Print and shaded views of the part. All mm, measured from the part's lowest x, y and z. A direction names the side the tool comes from. Round coordinates to 2 decimals unless told otherwise and drop trailing zeros. Loops run counter-clockwise (first coordinate to the right, second up) from the corner with the lowest first, then second, coordinate; pieces in that order, holes last. Notation, with made-up numbers: (-14.5, -27.75) - (5.5, -27.75) arc R15 cw to (5.5, -5.75) - close; hole circle Ø11 at (4.25, -33.75). An arc over 180 degrees is marked (long way). Use one line per item in the form item = value.
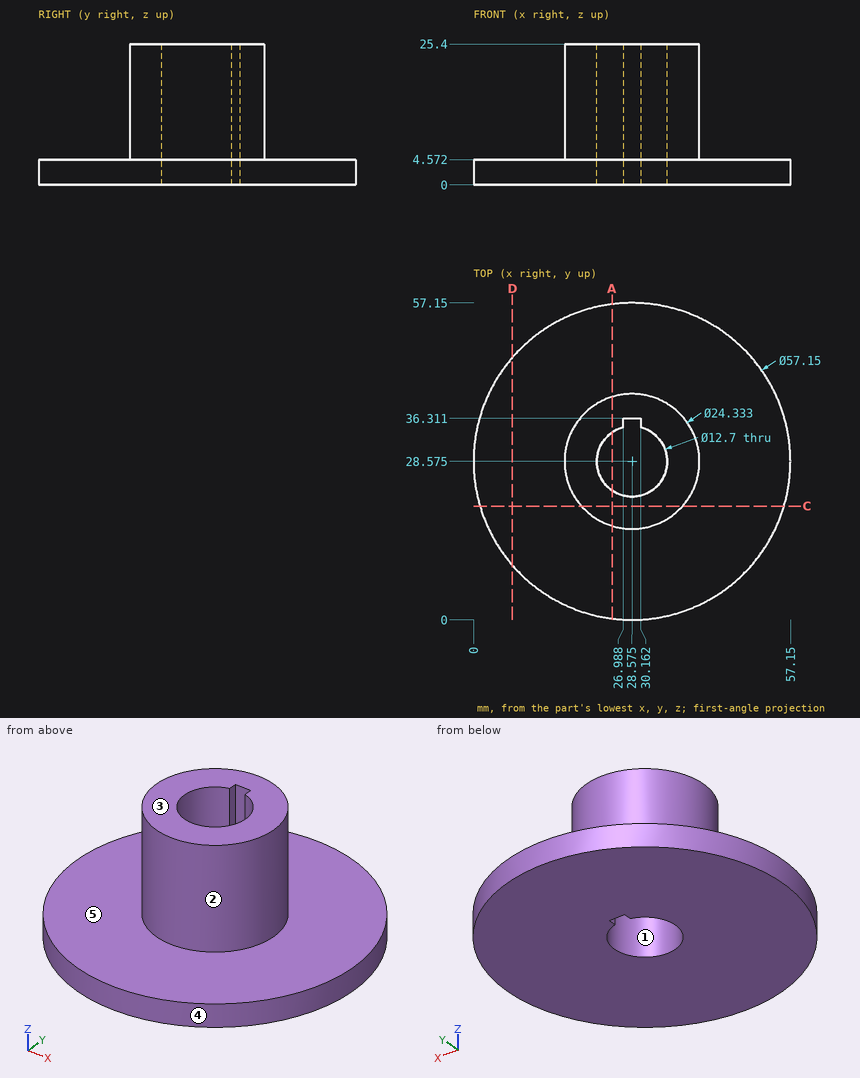
1. Cut at A-A, the plane x = 25. Give the cut face in (y, z) (1 decimal), plus the area to 3 significant figures.
Geometry check:
outline = (0.2, 0) - (23.3, 0) - (23.3, 25.4) - (16.9, 25.4) - (16.9, 4.6) - (0.2, 4.6) - close; (33.8, 0) - (56.9, 0) - (56.9, 4.6) - (40.2, 4.6) - (40.2, 25.4) - (33.8, 25.4) - close
area = 477 mm^2
2. Pull direction X, two halves, no side cores. Call the marked faces 1, 2 and 3: +X half, -X half, draft (parallel to the pull), parting line (faces both ways), or undercut.
Geometry check:
face_1 = undercut
face_2 = parting line
face_3 = draft
3. Flat gauge pins, fed straight in: pin 1 (3 mm diameter, centred on x = 22, z = 19.5, fed in from -Y); pin 2 (1.3 mm diameter, centred on y = 35.5, z = 8.5, fed in from +X); pin 3 (4 mm diameter, centred on y = 22, z = 4.5, fed in from +X). Where does each tip first touch, or does it go through?
Geometry check:
pin_1 = 17.52
pin_2 = 39
pin_3 = 56.78
4. Wall check: probe 1 along Z at (x, y) = (9, 42.5); probe 2 along X at (y, z) = (25, 17.75) (1 decimal); probe 3 along X at (y, z) = (29.5, 13.5). Give the ranges that are in metal, low to high.
Geometry check:
probe_1 = 0 to 4.57
probe_2 = 16.9 to 23.3, 33.8 to 40.2
probe_3 = 16.44 to 22.29, 34.86 to 40.71
5. Cut at C-C, the plane y = 20.5. Give the cut face in (x, z) (1 decimal), plus the area to 3 significant figures.
Geometry check:
outline = (1.2, 0) - (56, 0) - (56, 4.6) - (37.7, 4.6) - (37.7, 25.4) - (19.5, 25.4) - (19.5, 4.6) - (1.2, 4.6) - close
area = 630 mm^2
6. Cut at D-D, the plane x = 7. Give the cut face in (y, z), plus the area to 3 significant figures.
Geometry check:
outline = (9.84, 0) - (47.31, 0) - (47.31, 4.57) - (9.84, 4.57) - close
area = 171 mm^2
7. Tool access for the marked faces 4 and 5: list every direction of +Z, -Z, +X, -X, +Y, -Y with a clear straight run to the whole face (end or side of a thin tool).
Geometry check:
face_4 = +Z, -Z
face_5 = +Z
